Verification items for the finished model (mm, model axes). A direction names the side the tool comes from. Give positions to 0.01 mm unless a question says otherwise; leave off trailing zeros. Write each loop counter-clockwise with the first axis right and the second up, starting at its lowest first coordinate (ties: lowest second). Pieces come first, ordered by that corner, then holes. Notation, with made-up numbers: (88, 73.25) - (140, 73.25) arc R30 ccw to (140, 101.25) - close; hole circle Ø2 at (-13.75, 66.5). An arc over 180 degrees is marked (long way). Answer as a JSON object with one key per item and string values. Group by question number.
Item 1: Go/stop test with flat-tipped pins: pin 1 (10.5 mm diameter, centred on x = -52.15, z = 0, fed in from +Y); pin 2 (4.5 mm diameter, centred on y = 21.5, z = -68, fed in from +X); pin 3 (5 mm diameter, centred on x = 56.5, y = 22, fed in from -Z). Record where each tip stops, or that it passes through.
Item 2: Sectioned sample at D-D, the plane z = 58.5. Record the boundary of the cut face in (x, y).
Item 3: Tool access check on faces 1 (the face through (41, 21, -65.5)), 2 (the face through (41, 21, -70.838)), 3 (the face through (41, 21, 70.838)), 4 (the face through (-52, 3, 0)). Record the directions out of +Z, -Z, +X, -X, +Y, -Y that give a thin tool (end or side, any length) a straight path to the whole face; none if there is none.
Item 4: Sectioned sample at A-A, the plane y = 28. Record the boundary of the cut face in (x, z), and give its area (3 significant figures).
Item 5: Draft check along X on faces 5 (the face through (150, 5, 1)), 6 (the face through (-2, 10, -1)), 7 (the face through (-48.355, 6.549, 2.419)), 8 (the face through (-150, 5, 1)). Enter one of: +X half, -X half, draft (parallel to the pull), parting line (faces both ways), or undercut.
Item 6: Scan lines: line 1 along Z through (x, y) = (57, 15.5); line 2 along X through (y, z) = (5, 0); line 3 along Y through (x, z) = (129.5, 86). Record each from-to range of solid material in increasing order. Write a range as [from, to].
Item 7: Sectioned sample at B-B, the plane z = 0. Record the boundary of the cut face in (x, y), and give its area (3 significant figures).
Item 8: Sectioned sample at C-C, the plane x = 70. Record the boundary of the cut face in (y, z), and give its area (3 significant figures).
```python
from build123d import *

# Parameters (mm, degrees)
SKETCH1_W           = 300
SKETCH1_H           = 200
BOSS_EXTRUDE1_DEPTH = 10
SKETCH2_R           = 4.5
CUT_EXTRUDE1_DEPTH  = 7
SKETCH3_W           = 188.071582903
SKETCH3_H           = 5.337669468
BOSS_EXTRUDE2_DEPTH = 30


with BuildPart() as part:
    # Sketch1 → Boss-Extrude1 (new body)
    with BuildSketch(Plane(origin=(0, 0, 0), x_dir=(1, 0, 0), z_dir=(0, 1, 0))):
        Rectangle(SKETCH1_W, SKETCH1_H)
    extrude(amount=BOSS_EXTRUDE1_DEPTH)

    # Sketch2 → Cut-Extrude1 (cut)
    with BuildSketch(Plane(origin=(0, 10, 0), x_dir=(1, 0, 0), z_dir=(0, 1, 0))):
        with Locations(Location((-52.149355232, 0, 0), (0, 0, 270))):
            Circle(SKETCH2_R)
    extrude(amount=-CUT_EXTRUDE1_DEPTH, mode=Mode.SUBTRACT)

    # Sketch3 → Boss-Extrude2 (add)
    with BuildSketch(Plane(origin=(0, 3, 0), x_dir=(1, 0, 0), z_dir=(0, 1, 0))):
        with Locations((41.886436219, -68.168834734)):
            Rectangle(SKETCH3_W, SKETCH3_H)
        with Locations((41.886436219, 68.168834734)):
            Rectangle(SKETCH3_W, SKETCH3_H)
    extrude(amount=BOSS_EXTRUDE2_DEPTH)


solid = part.part
```
Geometry check:
{
 "1": {"pin 1": "y = 10", "pin 2": "x = 135.92", "pin 3": "z = -70.84"},
 "2": {"outline": "(-150, 0) - (150, 0) - (150, 10) - (-150, 10) - close"},
 "3": {"face 1": "+X, -X, +Y", "face 2": "-Z, +X, -X, +Y", "face 3": "+Z, +X, -X, +Y", "face 4": "+Y"},
 "4": {"outline": "(-52.15, -70.84) - (135.92, -70.84) - (135.92, -65.5) - (-52.15, -65.5) - close; (-52.15, 65.5) - (135.92, 65.5) - (135.92, 70.84) - (-52.15, 70.84) - close", "area": "2,010 mm^2"},
 "5": {"face 5": "+X half", "face 6": "draft", "face 7": "undercut", "face 8": "-X half"},
 "6": {"line 1": "[-70.84, -65.5], [65.5, 70.84]", "line 2": "[-150, -56.65], [-47.65, 150]", "line 3": "[0, 10]"},
 "7": {"outline": "(-150, 0) - (150, 0) - (150, 10) - (-47.65, 10) - (-47.65, 3) - (-56.65, 3) - (-56.65, 10) - (-150, 10) - close", "area": "2,940 mm^2"},
 "8": {"outline": "(0, -100) - (10, -100) - (10, -70.84) - (33, -70.84) - (33, -65.5) - (10, -65.5) - (10, 65.5) - (33, 65.5) - (33, 70.84) - (10, 70.84) - (10, 100) - (0, 100) - close", "area": "2,250 mm^2"}
}
